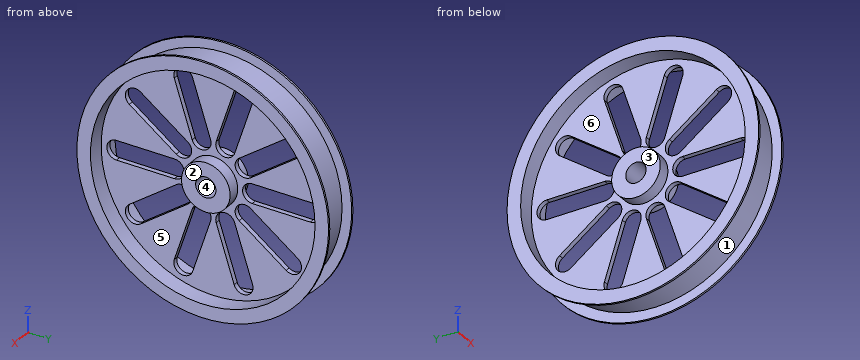
```python
from build123d import *

# Parameters (mm, degrees)
SKETCH3_R                = 13.335
CUT_EXTRUDE1_DEPTH       = 7.35
CUT_EXTRUDE1_DEPTH_BACK  = 45.45
CUT_EXTRUDE10_DEPTH      = 23.225
CUT_EXTRUDE10_DEPTH_BACK = 29.575


with BuildPart() as part:
    # Sketch2 → Revolve2 (revolve)
    with BuildSketch(Plane.XY):
        Polygon((22.86, 152.4), (-22.86, 152.4), (-22.86, 165.1), (-25.4, 165.1), (-25.4, 147.32), (-3.175, 147.32), (-3.175, 31.92334197), (-19.05, 31.92334197), (-19.05, 0), (19.05, 0), (19.05, 31.92334197), (3.175, 31.92334197), (3.175, 147.32), (25.4, 147.32), (25.4, 165.1), (22.86, 165.1), align=None)
    revolve(axis=Axis((217.873654092, 0, 0), (-1, 0, 0)))

    # Sketch3 → Cut-Extrude1 (cut, two sides)
    with BuildSketch(Plane.ZY.offset(19.05)) as cut_extrude1_sk:
        Circle(SKETCH3_R)
    extrude(amount=CUT_EXTRUDE1_DEPTH, mode=Mode.SUBTRACT)
    extrude(cut_extrude1_sk.sketch, amount=-CUT_EXTRUDE1_DEPTH_BACK, mode=Mode.SUBTRACT)

    # Sketch4 → Cut-Extrude10 (cut, two sides)
    with BuildSketch(Plane.ZY.offset(3.175)) as cut_extrude10_sk:
        with BuildLine():
            Line((12.7, 127.17334197), (12.7, 50.97334197))
            ThreePointArc((12.7, 50.97334197), (0, 38.27334197), (-12.7, 50.97334197))
            Line((-12.7, 50.97334197), (-12.7, 127.17334197))
            ThreePointArc((-12.7, 127.17334197), (0, 139.87334197), (12.7, 127.17334197))
        make_face()
        with BuildLine():
            Line((64.476099066, 110.350267589), (19.686862842, 48.703172618))
            ThreePointArc((19.686862842, 48.703172618), (22.496505966, 30.963784085), (40.235894499, 33.77342721))
            Line((40.235894499, 33.77342721), (85.025130723, 95.420522181))
            ThreePointArc((85.025130723, 95.420522181), (82.215487599, 113.159910714), (64.476099066, 110.350267589))
        make_face()
        with BuildLine():
            Line((117.024519751, 51.377141657), (44.55401321, 27.830046686))
            ThreePointArc((44.55401321, 27.830046686), (36.400111281, 11.8271131), (52.403044867, 3.673211172))
            Line((52.403044867, 3.673211172), (124.873551408, 27.220306143))
            ThreePointArc((124.873551408, 27.220306143), (133.027453337, 43.223239729), (117.024519751, 51.377141657))
        make_face()
        with BuildLine():
            Line((124.873551408, -27.220306143), (52.403044867, -3.673211172))
            ThreePointArc((52.403044867, -3.673211172), (36.400111281, -11.8271131), (44.55401321, -27.830046686))
            Line((44.55401321, -27.830046686), (117.024519751, -51.377141657))
            ThreePointArc((117.024519751, -51.377141657), (133.027453337, -43.223239729), (124.873551408, -27.220306143))
        make_face()
        with BuildLine():
            Line((85.025130723, -95.420522181), (40.235894499, -33.77342721))
            ThreePointArc((40.235894499, -33.77342721), (22.496505966, -30.963784085), (19.686862842, -48.703172618))
            Line((19.686862842, -48.703172618), (64.476099066, -110.350267589))
            ThreePointArc((64.476099066, -110.350267589), (82.215487599, -113.159910714), (85.025130723, -95.420522181))
        make_face()
        with BuildLine():
            Line((12.7, -127.17334197), (12.7, -50.97334197))
            ThreePointArc((12.7, -50.97334197), (0, -38.27334197), (-12.7, -50.97334197))
            Line((-12.7, -50.97334197), (-12.7, -127.17334197))
            ThreePointArc((-12.7, -127.17334197), (0, -139.87334197), (12.7, -127.17334197))
        make_face()
        with BuildLine():
            Line((-64.476099066, -110.350267589), (-19.686862842, -48.703172618))
            ThreePointArc((-19.686862842, -48.703172618), (-22.496505966, -30.963784085), (-40.235894499, -33.77342721))
            Line((-40.235894499, -33.77342721), (-85.025130723, -95.420522181))
            ThreePointArc((-85.025130723, -95.420522181), (-82.215487599, -113.159910714), (-64.476099066, -110.350267589))
        make_face()
        with BuildLine():
            Line((-117.024519751, -51.377141657), (-44.55401321, -27.830046686))
            ThreePointArc((-44.55401321, -27.830046686), (-36.400111281, -11.8271131), (-52.403044867, -3.673211172))
            Line((-52.403044867, -3.673211172), (-124.873551408, -27.220306143))
            ThreePointArc((-124.873551408, -27.220306143), (-133.027453337, -43.223239729), (-117.024519751, -51.377141657))
        make_face()
        with BuildLine():
            Line((-124.873551408, 27.220306143), (-52.403044867, 3.673211172))
            ThreePointArc((-52.403044867, 3.673211172), (-36.400111281, 11.8271131), (-44.55401321, 27.830046686))
            Line((-44.55401321, 27.830046686), (-117.024519751, 51.377141657))
            ThreePointArc((-117.024519751, 51.377141657), (-133.027453337, 43.223239729), (-124.873551408, 27.220306143))
        make_face()
        with BuildLine():
            Line((-85.025130723, 95.420522181), (-40.235894499, 33.77342721))
            ThreePointArc((-40.235894499, 33.77342721), (-22.496505966, 30.963784085), (-19.686862842, 48.703172618))
            Line((-19.686862842, 48.703172618), (-64.476099066, 110.350267589))
            ThreePointArc((-64.476099066, 110.350267589), (-82.215487599, 113.159910714), (-85.025130723, 95.420522181))
        make_face()
    extrude(amount=CUT_EXTRUDE10_DEPTH, mode=Mode.SUBTRACT)
    extrude(cut_extrude10_sk.sketch, amount=-CUT_EXTRUDE10_DEPTH_BACK, mode=Mode.SUBTRACT)


solid = part.part
```
Could you check a few things on this model? Use its own coordinates, in mm. Face numbers are marked on the shaded views. A direction names the side the tool comes from. Round coordinates to 2 decimals unless told otherwise and drop trailing zeros. Order: outer loops, then holes, each group sorted by start corner. A loop starts at its lowest first (then second) coordinate and runs counter-clockwise, first axis right, second up. Notation, with made-up numbers: (88, -22) -> (101, -22) arc R16 cw to (101, 1) -> close; hole circle Ø3 at (-36, 71.5). An arc over 180 degrees is marked (long way). One line per question, with ' | ' between items.
Q1. If I drill on line 1 (Y direction, x = 17, z = 0) (3 decimals); line 2 (Y direction, x = -20.75, z = 0); line 3 (Y direction, x = -2.5, z = 88), over which ranges is the centre line in solid material (lowest first)? Write a range as from..to.
Computed values:
line 1: -152.4..-147.32, -31.923..-13.335, 13.335..31.923, 147.32..152.4 | line 2: -152.4..-147.32, 147.32..152.4 | line 3: -124.43..-41.95, -15.24..15.24, 41.95..124.43
Q2. If we section it at C-C on z = -97.5: Write out the boundary of the cut face in (x, y) (3 decimals).
Computed values:
outline: (-25.4, -133.236) -> (-22.86, -133.236) -> (-22.86, -117.13) -> (22.86, -117.13) -> (22.86, -133.236) -> (25.4, -133.236) -> (25.4, -110.44) -> (3.175, -110.44) -> (3.175, -45.033) -> (-3.175, -45.033) -> (-3.175, -110.44) -> (-25.4, -110.44) -> close; (-25.4, 110.44) -> (-3.175, 110.44) -> (-3.175, 45.033) -> (3.175, 45.033) -> (3.175, 110.44) -> (25.4, 110.44) -> (25.4, 133.236) -> (22.86, 133.236) -> (22.86, 117.13) -> (-22.86, 117.13) -> (-22.86, 133.236) -> (-25.4, 133.236) -> close; (-3.175, -18.326) -> (3.175, -18.326) -> (3.175, 18.326) -> (-3.175, 18.326) -> close
Q3. Which directions (+Z, -Z, +X, -X, +Y, -Y) give clear straight access to the entire face, cutting with the end or side of a thin tool? Please do the marked faces 4, 5 and 6.
Computed values:
face 4: +X, -X | face 5: +X | face 6: -X
Q4. We'd pull the mould along X, two halves only. Please class the marked faces 1, 2 and 3: released by +X, released by -X, zero draft, split by the parting line, or undercut.
Computed values:
face 1: undercut | face 2: released by +X | face 3: released by -X
Q5. I'm going to push flat-ended pins straight in: pin 1 (6 mm diameter, centred on x = -7, z = 56, fed in from +Y); pin 2 (1.9 mm diameter, centred on x = 0, y = 76, fed in from +Z); pin 3 (1.5 mm diameter, centred on x = -6.5, z = -131.5, fed in from +Y). Where does each tip first touch, or does it pass through?
Computed values:
pin 1: y = 142.89 | pin 2: z = 132.64 | pin 3: y = 78.3
Q6. If we section it at A-A on y = -62.5: Give the number of separate pieces and of enclosed holes in the cut face, plus the area to 3 significant figures.
Computed values:
separate pieces: 4 | enclosed holes: 0 | area: 1,840 mm²
